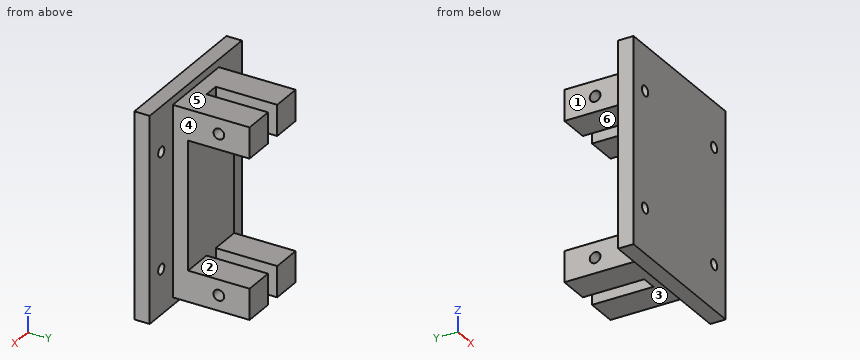
Autodesk Inventor part; units mm, degrees
ref_plane "YZ Plane" through (0, 0, 0) normal (1, 0, 0) x (0, 1, 0)
ref_plane "XZ Plane" through (0, 0, 0) normal (0, 1, 0) x (-1, 0, 0)
ref_plane "XY Plane" through (0, 0, 0) normal (0, 0, 1) x (1, 0, 0)
sketch "Sketch1" plane through (0, 0, 0) normal (0, 1, 0) x (-1, 0, 0)
  circle A0 centre (11.25, 11.25) radius 1
  circle A1 centre (11.25, -11.25) radius 1
  circle A2 centre (-11.25, 11.25) radius 1
  circle A3 centre (-11.25, -11.25) radius 1
  line L0 (-7.5, -18.5) -> (7.5, -18.5)
  line L1 (7.5, -18.5) -> (7.5, 18.5)
  line L2 (7.5, 18.5) -> (-7.5, 18.5)
  line L3 (-7.5, 18.5) -> (-7.5, -18.5)
  line L4 (-15, -20) -> (15, -20)
  line L5 (15, -20) -> (15, 20)
  line L6 (15, 20) -> (-15, 20)
  line L7 (-15, 20) -> (-15, -20)
  line L8 (7.5, -18.5) -> (1.5, -18.5)
  line L9 (1.5, -18.5) -> (1.5, -12.5)
  line L10 (1.5, -12.5) -> (7.5, -12.5)
  line L11 (7.5, -12.5) -> (7.5, -18.5)
  line L12 (-7.5, -18.5) -> (-1.5, -18.5)
  line L13 (-1.5, -18.5) -> (-1.5, -12.5)
  line L14 (-1.5, -12.5) -> (-7.5, -12.5)
  line L15 (-7.5, -12.5) -> (-7.5, -18.5)
  line L16 (-7.5, 18.5) -> (-1.5, 18.5)
  line L17 (-1.5, 18.5) -> (-1.5, 12.5)
  line L18 (-1.5, 12.5) -> (-7.5, 12.5)
  line L19 (-7.5, 12.5) -> (-7.5, 18.5)
  line L20 (7.5, 18.5) -> (1.5, 18.5)
  line L21 (1.5, 18.5) -> (1.5, 12.5)
  line L22 (1.5, 12.5) -> (7.5, 12.5)
  line L23 (7.5, 12.5) -> (7.5, 18.5)
  point P0 (0, 0)
extrude "Extrusion7" add sketch "Sketch1" along normal blind 18 contours L3 L14 L13 L0 | L9 L10 L1 L0 | L3 L2 L17 L18 | L22 L21 L2 L1
extrude "Extrusion8" add sketch "Sketch1" along normal blind 6 contours L13 L14 L3 L18 L17 L2 L21 L22 L1 L10 L9 L0
extrude "Extrusion9" add sketch "Sketch1" along normal blind 3
sketch "Sketch4" plane through (-7.5, 18, 12.5) normal (-1, 0, 0) x (0, 0, 1)
  line L0 (-25, -12) -> (-31, -12)
  line L1 (-28, -12) -> (-28, -6)
  line L2 (6, -12) -> (0, -12)
  line L3 (3, -12) -> (3, -6)
  circle A0 centre (-28, -6) radius 1.05
  circle A1 centre (3, -6) radius 1.05
  point P0 (-12.5, -18)
  dimension "d65" = 6
  dimension "d66" = 6
  dimension "d67" = 2.1
  dimension "d68" = 2.1
extrude "Extrusion10" cut sketch "Sketch4" against normal blind 18
properties part number "camera_plate2"
Part model, mm, in its own coordinate system. Face numbers are marked on the shaded views. A direction names the side the tool comes from. Coordinates: 2 decimals unless noted, no trailing zeros. Loops run counter-clockwise (first coordinate to the right, second up) from the corner with the lowest first, then second, coordinate; pieces in that order, holes last. Notation, with made-up numbers: M 49.25,64.25 L 77.25,64.25 A25 ccw 77.25,86.25 Z; hole C 80,48.25 d7. An arc over 180 degrees is marked long. Use a Markdown table: item, result. Add a question column.
Q1. Probe L1, parallel to Z at x = -5.3, y = 12; L2, parallel to Z at x = 11.25, y = 1.15; L3, parallel to Z at x = -6.75, y = 14.5. List the from-to ranges inside material, lowest first.
Q2. Which spindle directions (+Z, -Z, +X, -X, +Y, -Y) get a long thin tool onto all of the face, cutting with end or side? Do the marked faces 4, 5 and 6. Say none if no direction does.
Q3. Cut at C-C (y = 15.25). Write the cut outline in (x, z), and give its area (3 significant figures).
Q4. Pin check, flat tips, straight feed: P1, Ø5, axis at x = -5.5, y = 10.5, coming from the -Z side; P2, Ø1.8, axis at y = 13.5, z = -15, coming from the -X side; P3, Ø5, axis at y = 7.5, z = 14.5, coming from the +X side; P4, Ø1.7, axis at y = 12, z = -15.5, coming from the +X side. Stop position of each tip, or through.
Q5. Cut at B-B (x = -7). Write the cut outline in (y, z).
Q6. Mould opens along Z. For the marked faces 1, 2 and 3 say: +Z half, -Z half, draft (parallel to the pull), parting line (faces both ways), or undercut.
Q7. Cut at D-D (x = 11.25). Write the cut outline in (y, z), and give its area (3 significant figures).
Q8. Cut at A-A (z = -11.25). Write the cut outline in (x, y).
Worked out:
| question | item | result |
|---|---|---|
| 1 | L1 | z = -18.5 to -16.55, -14.45 to -12.5, 12.5 to 14.45, 16.55 to 18.5 |
| 1 | L2 | z = -20 to -12.25, -10.25 to 10.25, 12.25 to 20 |
| 1 | L3 | z = -18.5 to -12.5, 12.5 to 18.5 |
| 2 | face 4 | +Z, -Z, +X, +Y |
| 2 | face 5 | +Z, +X, -X, +Y |
| 2 | face 6 | +X, -X, +Y |
| 3 | outline | M -7.5,-18.5 L -1.5,-18.5 L -1.5,-12.5 L -7.5,-12.5 Z; M -7.5,12.5 L -1.5,12.5 L -1.5,18.5 L -7.5,18.5 Z; M 1.5,-18.5 L 7.5,-18.5 L 7.5,-12.5 L 1.5,-12.5 Z; M 1.5,12.5 L 7.5,12.5 L 7.5,18.5 L 1.5,18.5 Z |
| 3 | area | 144 mm2 |
| 4 | P1 | stops at z = -18.5 |
| 4 | P2 | stops at x = -7.5 |
| 4 | P3 | stops at x = 7.5 |
| 4 | P4 | passes through |
| 5 | outline | M 0,-20 L 3,-20 L 3,-18.5 L 18,-18.5 L 18,-12.5 L 6,-12.5 L 6,12.5 L 18,12.5 L 18,18.5 L 3,18.5 L 3,20 L 0,20 Z; hole C 12,-15.5 d2.1; hole C 12,15.5 d2.1 |
| 6 | face 1 | draft |
| 6 | face 2 | undercut |
| 6 | face 3 | -Z half |
| 7 | outline | M 0,-20 L 3,-20 L 3,-12.25 L 0,-12.25 Z; M 0,-10.25 L 3,-10.25 L 3,10.25 L 0,10.25 Z; M 0,12.25 L 3,12.25 L 3,20 L 0,20 Z |
| 7 | area | 108 mm2 |
| 8 | outline | M -15,0 L -12.25,0 L -12.25,3 L -15,3 Z; M -10.25,0 L 10.25,0 L 10.25,3 L 7.5,3 L 7.5,6 L -7.5,6 L -7.5,3 L -10.25,3 Z; M 12.25,0 L 15,0 L 15,3 L 12.25,3 Z |
